Autodesk Inventor part; units mm, degrees
ref_plane "Work Plane1" through (0, -1.7, 0) normal (0, 1, 0) x (1, 0, 0)
ref_plane "Work Plane2" through (0, -8, 0) normal (0, 1, 0) x (1, 0, 0)
ref_plane "YZ Plane" through (0, 0, 0) normal (1, 0, 0) x (0, 1, 0)
sketch "Sketch1" plane through (0, 0, 0) normal (0, 1, 0) x (-1, 0, 0)
  line L0 (0, 0) -> (24, 0)
  line L1 (24, 0) -> (24, -54)
  line L2 (24, -54) -> (0, -54)
  line L3 (0, -54) -> (0, 0)
  circle A0 centre (21.5, -9) radius 1.5
  circle A1 centre (2.5, -44) radius 1.5
  line L4 (24.5, -54.5) -> (24.5, 0.5)
  line L5 (24.5, 0.5) -> (-0.5, 0.5)
  line L6 (-0.5, 0.5) -> (-0.5, -54.5)
  line L7 (-0.5, -54.5) -> (24.5, -54.5)
  line L8 (29.5, 5.5) -> (29.5, -59.5)
  line L9 (29.5, -59.5) -> (-5.5, -59.5)
  line L10 (-5.5, -59.5) -> (-5.5, 5.5)
  line L11 (-5.5, 5.5) -> (29.5, 5.5)
  dimension "d0" = 24
  dimension "d1" = 54
  dimension "d2" = 3
  dimension "d3" = 3
  dimension "d4" = 9
  dimension "d5" = 2.5
  dimension "d6" = 2.5
  dimension "d7" = 10
  dimension "d8" = 0.5
  dimension "d9" = 5
extrude "Extrusion1" add sketch "Sketch1" against normal blind 1.7 contours L8 L9 L10 L11
ref_plane "Work Plane1" through (0, -1.7, 0) normal (0, 1, 0) x (1, 0, 0)
sketch "Sketch2" plane through (0, -1.7, 0) normal (0, 1, 0) x (1, 0, 0)
  line L0 (0, 0) -> (-24, 0)
  line L1 (-24, 0) -> (-24, 54)
  line L2 (-24, 54) -> (0, 54)
  line L3 (0, 54) -> (0, 0)
  circle A0 centre (-21.5, 9) radius 1.5
  circle A1 centre (-2.5, 44) radius 1.5
  line L4 (-24.5, 54.5) -> (-24.5, -0.5)
  line L5 (-24.5, -0.5) -> (0.5, -0.5)
  line L6 (0.5, -0.5) -> (0.5, 54.5)
  line L7 (0.5, 54.5) -> (-24.5, 54.5)
  line L8 (-29.5, -5.5) -> (-29.5, 59.5)
  line L9 (-29.5, 59.5) -> (5.5, 59.5)
  line L10 (5.5, 59.5) -> (5.5, -5.5)
  line L11 (5.5, -5.5) -> (-29.5, -5.5)
  circle A2 centre (-21.5, 9) radius 4
  circle A3 centre (-2.5, 44) radius 4
  point P0 (-24.5, 6.3542)
  point P1 (-24.5, 11.6458)
  point P2 (0.5, 46.6458)
  point P3 (0.5, 41.3542)
  dimension "d13" = 24
  dimension "d14" = 54
  dimension "d15" = 3
  dimension "d16" = 3
  dimension "d17" = 9
  dimension "d18" = 2.5
  dimension "d19" = 2.5
  dimension "d20" = 10
  dimension "d21" = 0.5
  dimension "d22" = 5
  dimension "d23" = 8
  dimension "d24" = 8
extrude "Extrusion2" add sketch "Sketch2" against normal blind 3 contours A3 L3 | L3 A3 L6 | A2 L4 L1 | L1 A2 | L6 A3 | A2 L4 | L8 L9 L10 L11
sketch "Sketch3" plane through (0, -4.7, 0) normal (0, -1, 0) x (1, 0, 0)
  line L0 (5.5, -59.5) -> (5.5, 5.5)
  line L1 (5.5, 5.5) -> (-29.5, 5.5)
  line L2 (-29.5, 5.5) -> (-29.5, -59.5)
  line L3 (-29.5, -59.5) -> (5.5, -59.5)
  point P0 (0, 0)
extrude "Extrusion3" add sketch "Sketch3" along normal blind 3.3
ref_plane "Work Plane2" through (0, -8, 0) normal (0, 1, 0) x (1, 0, 0)
sketch "Sketch4" plane through (0, -8, 0) normal (0, 1, 0) x (1, 0, 0)
  line L0 (-37, 2) -> (13, 2) construction
  line L1 (13, 2) -> (13, 52) construction
  line L2 (13, 52) -> (-37, 52) construction
  line L3 (-37, 52) -> (-37, 2) construction
  line L4 (0.5, -0.5) -> (-24.5, -0.5) construction
  line L5 (-12, -0.5) -> (-12, 54.5) construction
  line L6 (-24.5, 54.5) -> (0.5, 54.5) construction
  line L7 (-29.5, 59.5) -> (-29.5, -5.5)
  line L8 (-29.5, 27) -> (5.5, 27) construction
  line L9 (5.5, -5.5) -> (5.5, 59.5)
  circle A0 centre (-37, 2) radius 3
  circle A1 centre (-37, 52) radius 3
  circle A2 centre (13, 52) radius 3
  circle A3 centre (13, 2) radius 3
  circle A4 centre (-37, 2) radius 7.5
  line L10 (-29.5, -5.5) -> (5.5, -5.5)
  circle A5 centre (-37, 52) radius 7.5
  circle A6 centre (13, 52) radius 7.5
  circle A7 centre (13, 2) radius 7.5
  line L11 (5.5, 59.5) -> (-29.5, 59.5)
  line L12 (5.5, -5.5) -> (13, -5.5)
  line L13 (5.5, 59.5) -> (13, 59.5)
  line L14 (13, 44.5) -> (5.5, 44.5)
  line L15 (13, 9.5) -> (5.5, 9.5)
  line L16 (-29.5, -5.5) -> (-37, -5.5)
  line L17 (-37, 9.5) -> (-29.5, 9.5)
  line L18 (-37, 44.5) -> (-29.5, 44.5)
  line L19 (-37, 59.5) -> (-29.5, 59.5)
  point P0 (0, 0)
  dimension "d30" = 50
  dimension "d31" = 50
  dimension "d32" = 25
  dimension "d33" = 25
  dimension "d34" = 6
  dimension "d35" = 6
  dimension "d36" = 6
  dimension "d37" = 6
extrude "Extrusion4" add sketch "Sketch4" along normal blind 4 contours L7 A5 L19 | A5 | L7 L18 A5 | L13 A6 L9 | A6 L14 L9 | A6 | L7 A4 L17 | A4 | L7 L16 A4 | L15 A7 L9 | A7 L12 L9 | A7
fillet "Fillet1" radius 4 6 edges at (5.5, -2.85, -59.5) (5.5, -0.85, -59.5) (-29.5, -2, -59.5) (-29.5, -2, 5.5) (5.5, -0.85, 5.5) (5.5, -2.85, 5.5)
chamfer "Chamfer1" distance 1.5 angle 45 2 edges at (-4, -1.7, -44) (-23, -1.7, -9)
sketch "Sketch5" plane through (-2.5, -4.7, -44) normal (0, 1, 0) x (1, 0, 0)
  circle A0 centre (-19, -35) radius 1.5
  circle A1 centre (0, 0) radius 1.5
  point P0 (2.5, -44)
extrude "Extrusion5" cut sketch "Sketch5" against normal through all
sketch "Sketch6" plane through (0, 0, 0) normal (0, 1, 0) x (1, 0, 0)
  line L0 (-24.5, 54.5) -> (0.5, 54.5)
  line L1 (0.5, 54.5) -> (0.5, 59.563)
  line L2 (1.5, 59.5) -> (-25.5, 59.5)
  line L3 (-24.5, 54.5) -> (-24.5, 59.5)
  line L4 (0.5, -0.5) -> (-24.5, -0.5)
  line L5 (0.5, -0.5) -> (0.5, -5.5)
  line L6 (-25.5, -5.5) -> (1.5, -5.5)
  line L7 (-24.5, -0.5) -> (-24.5, -5.5)
  point P0 (0, 0)
  point P1 (0.5, 59.5)
extrude "Extrusion6" cut sketch "Sketch6" against normal up to surface (4.7 mm away)
equation "\"d3\" = d2"
equation "\"d6\" = d5"
equation "\"d16\" = d15"
equation "\"d19\" = d18"
equation "\"d24\" = d23"
equation "\"d32\" = 0.5 * d30"
equation "\"d33\" = 0.5 * d31"
equation "\"d35\" = d34"
equation "\"d36\" = d34"
equation "\"d37\" = d34"
properties part number "DCDC Converter Mount"
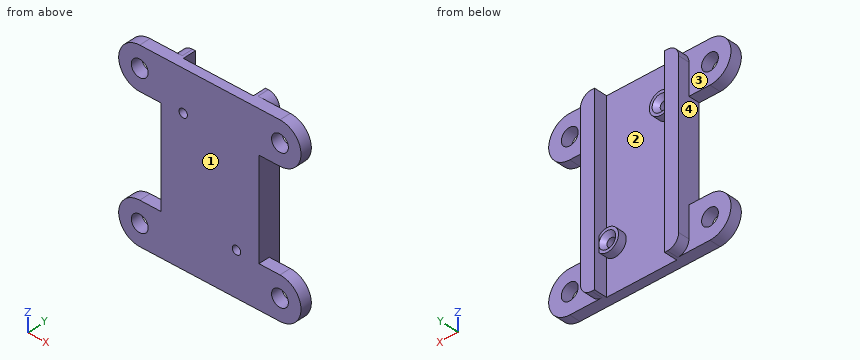
The model under review builds one solid part; all positions refer to its coordinate system, in mm. Face numbers are marked on the shaded views. A direction names the side the tool comes from. Round coordinates to 2 decimals unless told otherwise and drop trailing zeros. Order: outer loops, then holes, each group sorted by start corner. A loop starts at its lowest first (then second) coordinate and runs counter-clockwise, first axis right, second up. Notation, with made-up numbers: (89, 10) -> (126, 10) arc R30 cw to (126, 34) -> close; hole circle Ø11 at (28, -2). An arc over 180 degrees is marked (long way). One line per item, written item: value. Start each with the question number.
Q1. Take a section at D-D (x = -21.5). Write out the cut boundary in (y, z), and give its area (3 significant figures).
Q2. Take a section at B-B (z = -2). Write out the cut boundary in (x, y).
Q3. Take a section at A-A (x = -32). Write out the cut boundary in (y, z), and give its area (3 significant figures).
Q4. Clearance check with flat-ended pins moving along their axes: pin 1 Ø5.5 at (x, z) = (-20.5, -7.5) entering from +Y; pin 2 Ø12.5 at (x, z) = (-13.5, -37.5) entering from +Y; pin 3 Ø7.5 at (x, z) = (10.5, -1) entering from +Y. State where each tip first meets the part, or that it passes through.
Q5. Mouldability with a two-part tool opening along Z and no side actions: class the marked faces 3 and 4 as released by +Z, released by -Z, zero draft, split by the parting line, or undercut.
Q6. Wall thickness on line 1 (X direction, y = -6.6, z = -52); line 2 (Z direction, x = 13, y = -5.85); line 3 (X direction, y = -6, z = -44): over which ranges is each line inside the solid? List them lowest first.
Q7. Machinability: for the marked faces 1 and 2, which of the approach directions +Z, -Z, +X, -X, +Y, -Y give a long, thin tool a straight path to every point of the face, cutting with its end or side? Answer none if there is none.
Q8. Take a section at C-C (z = -29.5). Write out the cut boundary in (x, y), and give its area (4 significant figures).
Reported:
1. outline: (-8, -59.5) -> (-4.7, -59.5) -> (-4.7, -13) -> (-1.7, -13) -> (-1.7, -12) -> (-3.2, -10.5) -> (-8, -10.5) -> close; (-8, -7.5) -> (-3.2, -7.5) -> (-1.7, -6) -> (-1.7, -5) -> (-4.7, -5) -> (-4.7, 5.5) -> (-8, 5.5) -> close
1. area: 217 mm2
2. outline: (-44.5, -8) -> (-40, -8) -> (-40, -4) -> (-44.5, -4) -> close; (-34, -8) -> (10, -8) -> (10, -4) -> (5.5, -4) -> (5.5, 0) -> (0.5, 0) -> (0.5, -4.7) -> (-24.5, -4.7) -> (-24.5, 0) -> (-29.5, 0) -> (-29.5, -4) -> (-34, -4) -> close; (16, -8) -> (20.5, -8) -> (20.5, -4) -> (16, -4) -> close
3. outline: (-8, -59.5) -> (-4, -59.5) -> (-4, -44.5) -> (-8, -44.5) -> close; (-8, -9.5) -> (-4, -9.5) -> (-4, 5.5) -> (-8, 5.5) -> close
3. area: 120 mm2
4. pin 1: stops at y = -1.7
4. pin 2: stops at y = -4.7
4. pin 3: stops at y = -4
5. face 3: zero draft
5. face 4: undercut
6. line 1: x = -44.5 to -40, -34 to 10, 16 to 20.5
6. line 2: z = -59.5 to -55, -49 to -44.5, -9.5 to -5, 1 to 5.5
6. line 3: x = -29.5 to -4, -1 to 5.5
7. face 1: +Z, -Z, +X, -X, -Y
7. face 2: +Y
8. outline: (-29.5, -8) -> (5.5, -8) -> (5.5, 0) -> (0.5, 0) -> (0.5, -4.7) -> (-24.5, -4.7) -> (-24.5, 0) -> (-29.5, 0) -> close
8. area: 162.5 mm2
